from build123d import *

# Parameters (mm, degrees)
F1_DEPTH = 1.5
F2_DEPTH = 2
F3_DEPTH = 11


with BuildPart() as f1:
    # F0 (on Top) → F1 (new body)
    with BuildSketch(Plane.XY):
        with BuildLine():
            ThreePointArc((10, 30.4), (-2.588190451, 40.0592582629), (-8.6602540378, 25.4))
            Line((-8.6602540378, 25.4), (-4.2868257487, 27.925))
            ThreePointArc((-4.2868257487, 27.925), (-1.2811542733, 35.1813328401), (4.95, 30.4))
            ThreePointArc((4.95, 30.4), (4.7813328401, 29.1188457267), (4.2868257487, 27.925))
            Line((4.2868257487, 27.925), (8.6602540378, 25.4))
            ThreePointArc((8.6602540378, 25.4), (9.6592582629, 27.811809549), (10, 30.4))
        make_face()
        with BuildLine():
            Line((0, 25.45), (0, 20.4))
            ThreePointArc((0, 20.4), (5, 21.7397459622), (8.6602540378, 25.4))
            Line((8.6602540378, 25.4), (4.2868257487, 27.925))
            ThreePointArc((4.2868257487, 27.925), (2.475, 26.1131742513), (0, 25.45))
        make_face()
        with BuildLine():
            ThreePointArc((-8.6602540378, 25.4), (-5, 21.7397459622), (0, 20.4))
            Line((0, 20.4), (0, 25.45))
            ThreePointArc((0, 25.45), (-2.475, 26.1131742513), (-4.2868257487, 27.925))
            Line((-4.2868257487, 27.925), (-8.6602540378, 25.4))
        make_face()
        with BuildLine():
            ThreePointArc((8.6602540378, 25.4), (5, 21.7397459622), (0, 20.4))
            ThreePointArc((0, 20.4), (-5, 21.7397459622), (-8.6602540378, 25.4))
            ThreePointArc((-8.6602540378, 25.4), (-10.5489683598, 6.0904497222), (-26.327172275, -5.2))
            ThreePointArc((-26.327172275, -5.2), (-19.2561044632, -8.1289321881), (-16.327172275, -15.2))
            ThreePointArc((-16.327172275, -15.2), (-16.6679140122, -17.788190451), (-17.6669182372, -20.2))
            ThreePointArc((-17.6669182372, -20.2), (0, -12.1808994444), (17.6669182372, -20.2))
            ThreePointArc((17.6669182372, -20.2), (17.6669182372, -10.2), (26.327172275, -5.2))
            ThreePointArc((26.327172275, -5.2), (10.5489683598, 6.0904497222), (8.6602540378, 25.4))
        make_face()
        with BuildLine():
            ThreePointArc((0, 10), (7.0710678119, 7.0710678119), (10, 0))
            ThreePointArc((10, 0), (-7.0710678119, -7.0710678119), (0, 10))
        make_face(mode=Mode.SUBTRACT)
        with BuildLine():
            ThreePointArc((-16.327172275, -15.2), (-19.2561044632, -8.1289321881), (-26.327172275, -5.2))
            Line((-26.327172275, -5.2), (-26.327172275, -10.25))
            ThreePointArc((-26.327172275, -10.25), (-22.8269937082, -11.6998214331), (-21.377172275, -15.2))
            ThreePointArc((-21.377172275, -15.2), (-21.5458394349, -16.4811542733), (-22.0403465263, -17.675))
            Line((-22.0403465263, -17.675), (-17.6669182372, -20.2))
            ThreePointArc((-17.6669182372, -20.2), (-16.6679140122, -17.788190451), (-16.327172275, -15.2))
        make_face()
        with BuildLine():
            Line((-26.327172275, -10.25), (-26.327172275, -5.2))
            ThreePointArc((-26.327172275, -5.2), (-34.9874263129, -20.2), (-17.6669182372, -20.2))
            Line((-17.6669182372, -20.2), (-22.0403465263, -17.675))
            ThreePointArc((-22.0403465263, -17.675), (-30.6139980238, -17.675), (-26.327172275, -10.25))
        make_face()
        with BuildLine():
            ThreePointArc((36.327172275, -15.2), (33.3982400869, -8.1289321881), (26.327172275, -5.2))
            Line((26.327172275, -5.2), (26.327172275, -10.25))
            ThreePointArc((26.327172275, -10.25), (29.8273508419, -11.6998214331), (31.277172275, -15.2))
            ThreePointArc((31.277172275, -15.2), (27.6083265483, -19.9813328401), (22.0403465263, -17.675))
            Line((22.0403465263, -17.675), (17.6669182372, -20.2))
            ThreePointArc((17.6669182372, -20.2), (28.9153627261, -24.8592582629), (36.327172275, -15.2))
        make_face()
        with BuildLine():
            Line((26.327172275, -10.25), (26.327172275, -5.2))
            ThreePointArc((26.327172275, -5.2), (17.6669182372, -10.2), (17.6669182372, -20.2))
            Line((17.6669182372, -20.2), (22.0403465263, -17.675))
            ThreePointArc((22.0403465263, -17.675), (22.0403465263, -12.725), (26.327172275, -10.25))
        make_face()
    extrude(amount=F1_DEPTH)

    # F0 (on Top) → F2 (join)
    with BuildSketch(Plane.XY):
        with BuildLine():
            ThreePointArc((4.95, 30.4), (-1.2811542733, 35.1813328401), (-4.2868257487, 27.925))
            Line((-4.2868257487, 27.925), (-3.4208003449, 28.425))
            ThreePointArc((-3.4208003449, 28.425), (-1.0223352282, 34.2154070138), (3.95, 30.4))
            ThreePointArc((3.95, 30.4), (3.8154070138, 29.3776647718), (3.4208003449, 28.425))
            Line((3.4208003449, 28.425), (4.2868257487, 27.925))
            ThreePointArc((4.2868257487, 27.925), (4.7813328401, 29.1188457267), (4.95, 30.4))
        make_face()
        with BuildLine():
            ThreePointArc((-4.2868257487, 27.925), (-2.475, 26.1131742513), (0, 25.45))
            Line((0, 25.45), (0, 26.45))
            ThreePointArc((0, 26.45), (-1.975, 26.9791996551), (-3.4208003449, 28.425))
            Line((-3.4208003449, 28.425), (-4.2868257487, 27.925))
        make_face()
        with BuildLine():
            Line((0, 26.45), (0, 25.45))
            ThreePointArc((0, 25.45), (2.475, 26.1131742513), (4.2868257487, 27.925))
            Line((4.2868257487, 27.925), (3.4208003449, 28.425))
            ThreePointArc((3.4208003449, 28.425), (1.975, 26.9791996551), (0, 26.45))
        make_face()
        with BuildLine():
            Line((26.327172275, -11.25), (26.327172275, -10.25))
            ThreePointArc((26.327172275, -10.25), (22.0403465263, -12.725), (22.0403465263, -17.675))
            Line((22.0403465263, -17.675), (22.9063719301, -17.175))
            ThreePointArc((22.9063719301, -17.175), (22.9063719301, -13.225), (26.327172275, -11.25))
        make_face()
        with BuildLine():
            ThreePointArc((31.277172275, -15.2), (29.8273508419, -11.6998214331), (26.327172275, -10.25))
            Line((26.327172275, -10.25), (26.327172275, -11.25))
            ThreePointArc((26.327172275, -11.25), (29.1202440607, -12.4069282143), (30.277172275, -15.2))
            ThreePointArc((30.277172275, -15.2), (27.3495075032, -19.0154070138), (22.9063719301, -17.175))
            Line((22.9063719301, -17.175), (22.0403465263, -17.675))
            ThreePointArc((22.0403465263, -17.675), (27.6083265483, -19.9813328401), (31.277172275, -15.2))
        make_face()
        with BuildLine():
            Line((-26.327172275, -11.25), (-26.327172275, -10.25))
            ThreePointArc((-26.327172275, -10.25), (-30.6139980238, -17.675), (-22.0403465263, -17.675))
            Line((-22.0403465263, -17.675), (-22.9063719301, -17.175))
            ThreePointArc((-22.9063719301, -17.175), (-29.74797262, -17.175), (-26.327172275, -11.25))
        make_face()
        with BuildLine():
            ThreePointArc((-21.377172275, -15.2), (-22.8269937082, -11.6998214331), (-26.327172275, -10.25))
            Line((-26.327172275, -10.25), (-26.327172275, -11.25))
            ThreePointArc((-26.327172275, -11.25), (-23.5341004894, -12.4069282143), (-22.377172275, -15.2))
            ThreePointArc((-22.377172275, -15.2), (-22.5117652612, -16.2223352282), (-22.9063719301, -17.175))
            Line((-22.9063719301, -17.175), (-22.0403465263, -17.675))
            ThreePointArc((-22.0403465263, -17.675), (-21.5458394349, -16.4811542733), (-21.377172275, -15.2))
        make_face()
    extrude(amount=F2_DEPTH)

    # F0 (on Top) → F3 (join)
    with BuildSketch(Plane.XY):
        with BuildLine():
            Line((-3.4208003449, 28.425), (0, 30.4))
            Line((0, 30.4), (3.4208003449, 28.425))
            ThreePointArc((3.4208003449, 28.425), (3.8154070138, 29.3776647718), (3.95, 30.4))
            ThreePointArc((3.95, 30.4), (-1.0223352282, 34.2154070138), (-3.4208003449, 28.425))
        make_face()
        with BuildLine():
            ThreePointArc((-3.4208003449, 28.425), (-1.975, 26.9791996551), (0, 26.45))
            Line((0, 26.45), (0, 30.4))
            Line((0, 30.4), (-3.4208003449, 28.425))
        make_face()
        with BuildLine():
            Line((0, 30.4), (0, 26.45))
            ThreePointArc((0, 26.45), (1.975, 26.9791996551), (3.4208003449, 28.425))
            Line((3.4208003449, 28.425), (0, 30.4))
        make_face()
        with BuildLine():
            ThreePointArc((-22.377172275, -15.2), (-23.5341004894, -12.4069282143), (-26.327172275, -11.25))
            Line((-26.327172275, -11.25), (-26.327172275, -15.2))
            Line((-26.327172275, -15.2), (-22.9063719301, -17.175))
            ThreePointArc((-22.9063719301, -17.175), (-22.5117652612, -16.2223352282), (-22.377172275, -15.2))
        make_face()
        with BuildLine():
            Line((-26.327172275, -15.2), (-26.327172275, -11.25))
            ThreePointArc((-26.327172275, -11.25), (-29.74797262, -17.175), (-22.9063719301, -17.175))
            Line((-22.9063719301, -17.175), (-26.327172275, -15.2))
        make_face()
        with BuildLine():
            Line((26.327172275, -15.2), (26.327172275, -11.25))
            ThreePointArc((26.327172275, -11.25), (22.9063719301, -13.225), (22.9063719301, -17.175))
            Line((22.9063719301, -17.175), (26.327172275, -15.2))
        make_face()
        with BuildLine():
            ThreePointArc((30.277172275, -15.2), (29.1202440607, -12.4069282143), (26.327172275, -11.25))
            Line((26.327172275, -11.25), (26.327172275, -15.2))
            Line((26.327172275, -15.2), (22.9063719301, -17.175))
            ThreePointArc((22.9063719301, -17.175), (27.3495075032, -19.0154070138), (30.277172275, -15.2))
        make_face()
    extrude(amount=F3_DEPTH)


solid = f1.part
The listing builds one solid part. Answer for the finished solid, in the listing's coordinates (mm). A direction names the side the tool comes from. Round coordinates to 2 decimals unless told otherwise and drop trailing zeros. Write each loop counter-clockwise with the first axis right and the second up, starting at its lowest first coordinate (ties: lowest second). Pieces come first, ordered by that corner, then holes. Notation, with made-up numbers: M -3.75,66 L 10.25,66 A34 ccw 10.25,105 Z; hole C 87.5,84 d9. An arc over 180 degrees is marked long. Write each question's results on one line, items separated by ' | '. Start each with the question number.
Item 1: Flat-ended cylindrical pins translate along their axes: pin 1 Ø6 at (x, z) = (20.5, 9) entering from +Y; pin 2 Ø4 at (y, z) = (27.5, 6) entering from +X; pin 3 Ø3 at (x, y) = (-8, -14) entering from +Z; pin 4 Ø3 at (x, z) = (16.5, 4.5) entering from +Y. Find the tip coordinate at first contact, or state that the pin passes through.
Item 2: For faces 1 (the face through (-4, 29, 2)), 2 (the face through (-35.13, -19.944, 0.74)), determine the directions among +Z, -Z, +X, -X, +Y, -Y from which every point of the face is accessible in a straight line to the end or side of a thin tool.
Item 3: A cutting plane is placed at B-B on y = 11. Write down the section's boundary in (x, z).
Item 4: A cutting plane is placed at C-C on x = -16. Write down the section's boundary in (y, z), and give its area (3 significant figures).
Item 5: For a pull along X with two mould halves and no side action, classify faces 3 (the face through (-6, -9, 0)), 4 (the face through (-0.2, 10.2, 1.5)), 5 (the face through (-10.41, 6.334, 0.74)), 6 (the face through (10.69, 5.85, 0.74)) as pulls with the +X half, pulls with the -X half, needs draft (parallel to the pull), parting line crosses it, or undercut.
Item 6: Straight lines are drawn through the part: L1, parallel to Y at x = 0, z = 1.05; L2, parallel to Z at x = 12.5, y = -12; L3, parallel to X at y = 0, z = 1.05. For each, find the intervals that lie inside material, in ascending order. Write a range as [from, to].
Item 7: A cutting plane is placed at A-A on z = 10. Write down the section's boundary in (x, y) (3 decimals).
Check sheet entries:
1) pin 1: y = -12.44 | pin 2: x = 3.85 | pin 3: z = 1.5 | pin 4: through
2) face 1: +Z | face 2: +Z, -Z
3) outline: M -8.42,0 L 8.42,0 L 8.42,1.5 L -8.42,1.5 Z
4) outline: M -18.48,0 L -0.33,0 L -0.33,1.5 L -18.48,1.5 Z | area: 27.2 mm²
5) face 3: needs draft | face 4: undercut | face 5: pulls with the -X half | face 6: pulls with the +X half
6) L1: [-12.18, -10], [10, 40.4] | L2: [0, 1.5] | L3: [-15.61, -10], [10, 15.61]
7) outline: C -26.327,-15.2 d7.9; C 0,30.4 d7.9; C 26.327,-15.2 d7.9
